Can you work these out from the model? Positions are in its coordinate system, mm. A direction names the side the tool comes from. Coordinates: 2 decimals unless noted, no trailing zeros. Order: outer loops, then holes, each group sorted by start corner. A loop starts at its lowest first (then second) coordinate and runs counter-clockwise, first axis right, second up. Notation, with made-up numbers: M -20.5,24.25 L 37.5,24.25 A28 cw 37.5,62.25 Z; hole C -13,29.25 d10. An arc over 180 degrees is marked long. Answer as CSV lines item,"result". Start each with the question number.
1. If we section it at C-C (y = -11): List the corners of the cut face in (x, z) for me, plus the area to 3 significant figures.
2. If we section it at B-B (x = 0): List the corners of the cut face in (y, z) for me.
3. If we section it at D-D (x = 18.4): List the corners of the cut face in (y, z) for me, plus the area to 3 significant figures.
4. I need wall thicknesses on line 1 along Z through (x, y) = (0, -6.15); line 2 along X through (y, z) = (-5.75, 5.25); line 3 along Y through (x, z) = (-18.5, 5). Which ranges of each line are inside material? Lowest first, please. Write a range as from..to.
5. Will these pins go through, and if not, where does the flat tip stop? pin 1 (6 mm diameter, centred on x = -18.4, z = 0, fed in from -Y); pin 2 (10.5 mm diameter, centred on x = 15, z = 4, fed in from -Y); pin 3 (4.5 mm diameter, centred on x = 18.4, z = 0, fed in from -Y); pin 4 (1 mm diameter, centred on y = -3.5, z = 1.5, fed in from -X).
6. If we section it at A-A (y = -6): List the corners of the cut face in (x, z) for me.
7. If we mould it in two halves opening along X, with no side actions, what happens to faces 3 (the face through (8.44, -8.2, -8.44)), 4 (the face through (13.4, -3.9, 0.1)), 5 (the face through (13.34, -2.071, 8.245))? For each: released by +X, released by -X, zero draft, split by the parting line, or undercut.
8. On a 3-axis mill with a long thin cutter (end or side, diameter ignored), from which of +Z, -Z, +X, -X, +Y, -Y can I reach the whole of each face in a straight line? I mean faces 1 (the face through (5.19, -5.93, -9.98)), 2 (the face through (-21, -2, 0)). Say none if no direction works.
```python
from build123d import *

# Parameters (mm, degrees)
F0_R     = 2.6
F0_R_2   = 4
F1_DEPTH = 4.2
F2_R     = 14.25
F2_R_2   = 13.25
F3_DEPTH = 0.3
F4_R     = 6.2
F4_R_2   = 4
F5_DEPTH = 7.8
F4_R_3   = 11.25
F6_DEPTH = 4
F7_SIZE  = 0.5


with BuildPart() as f1:
    # F0 (on Front) → F1 (new body)
    with BuildSketch(Plane.XZ):
        with BuildLine():
            ThreePointArc((-5.796875, -11.9146439407), (-13.25, 0), (-5.796875, 11.9146439407))
            Line((-5.796875, 11.9146439407), (-20.675, 4.6759357352))
            ThreePointArc((-20.675, 4.6759357352), (-23.6, 0), (-20.675, -4.6759357352))
            Line((-20.675, -4.6759357352), (-5.796875, -11.9146439407))
        make_face()
        with Locations((-18.4, 0)):
            Circle(F0_R, mode=Mode.SUBTRACT)
        with BuildLine():
            ThreePointArc((5.796875, -11.9146439407), (11.2332340346, -7.026873638), (13.25, 0))
            ThreePointArc((13.25, 0), (11.2332340346, 7.026873638), (5.796875, 11.9146439407))
            ThreePointArc((5.796875, 11.9146439407), (0, 13.25), (-5.796875, 11.9146439407))
            ThreePointArc((-5.796875, 11.9146439407), (-13.25, 0), (-5.796875, -11.9146439407))
            ThreePointArc((-5.796875, -11.9146439407), (0, -13.25), (5.796875, -11.9146439407))
        make_face()
        Circle(F0_R_2, mode=Mode.SUBTRACT)
        with BuildLine():
            ThreePointArc((5.796875, 11.9146439407), (11.2332340346, 7.026873638), (13.25, 0))
            ThreePointArc((13.25, 0), (11.2332340346, -7.026873638), (5.796875, -11.9146439407))
            Line((5.796875, -11.9146439407), (20.675, -4.6759357352))
            ThreePointArc((20.675, -4.6759357352), (23.6, 0), (20.675, 4.6759357352))
            Line((20.675, 4.6759357352), (5.796875, 11.9146439407))
        make_face()
        with Locations((18.4, 0)):
            Circle(F0_R, mode=Mode.SUBTRACT)
    extrude(amount=F1_DEPTH)

    # F2 (on face) → F3 (cut)
    with BuildSketch(Plane.XZ.offset(4.2)):
        Circle(F2_R)
        Circle(F2_R_2, mode=Mode.SUBTRACT)
    extrude(amount=-F3_DEPTH, mode=Mode.SUBTRACT)

    # F4 (on face) → F5 (join)
    with BuildSketch(Plane.XZ.offset(4.2)):
        Circle(F4_R)
        Circle(F4_R_2, mode=Mode.SUBTRACT)
    extrude(amount=F5_DEPTH)

    # F4 (on face) → F6 (join)
    with BuildSketch(Plane.XZ.offset(4.2)):
        with BuildLine():
            ThreePointArc((5.796875, -11.9146439407), (11.2332340346, -7.026873638), (13.25, 0))
            ThreePointArc((13.25, 0), (11.2332340346, 7.026873638), (5.796875, 11.9146439407))
            ThreePointArc((5.796875, 11.9146439407), (0, 13.25), (-5.796875, 11.9146439407))
            ThreePointArc((-5.796875, 11.9146439407), (-13.25, 0), (-5.796875, -11.9146439407))
            ThreePointArc((-5.796875, -11.9146439407), (0, -13.25), (5.796875, -11.9146439407))
        make_face()
        Circle(F4_R_3, mode=Mode.SUBTRACT)
    extrude(amount=F6_DEPTH)

    # F7
    f7_edges = [f1.edges().sort_by_distance(p)[0] for p in [
        (-4, -12, 0),
        (-6.2, -12, 0),
        (-11.25, -8.2, 0),
        (5.796875, -8.2, -11.914644),
    ]]
    chamfer(f7_edges, length=F7_SIZE)


solid = f1.part
```
Solved:
1,outline,"C 0,0 d12.4; hole C 0,0 d8"
1,area,"70.5 mm²"
2,outline,"M -12,-5.7 L -11.5,-6.2 L -4.2,-6.2 L -4.2,-11.25 L -7.7,-11.25 L -8.2,-11.75 L -8.2,-12.75 L -7.7,-13.25 L 0,-13.25 L 0,-4 L -11.5,-4 L -12,-4.5 Z; M -12,4.5 L -11.5,4 L 0,4 L 0,13.25 L -7.7,13.25 L -8.2,12.75 L -8.2,11.75 L -7.7,11.25 L -4.2,11.25 L -4.2,6.2 L -11.5,6.2 L -12,5.7 Z"
3,outline,"M -4.2,-5.78 L 0,-5.78 L 0,-2.6 L -4.2,-2.6 Z; M -4.2,2.6 L 0,2.6 L 0,5.78 L -4.2,5.78 Z"
3,area,"26.7 mm²"
4,line 1,"-13.25..-11.25, -6.2..-4, 4..6.2, 11.25..13.25"
4,line 2,"-12.17..-9.95, -3.3..3.3, 9.95..12.17"
4,line 3,"-4.2..0"
5,pin 1,"y = -4.2"
5,pin 2,"y = -8.2"
5,pin 3,"through"
5,pin 4,"x = -23.5"
6,outline,"C 0,0 d26.5; C 0,0 d12.4; hole C 0,0 d22.5; hole C 0,0 d8"
7,face 3,"zero draft"
7,face 4,"undercut"
7,face 5,"released by +X"
8,face 1,"-Y"
8,face 2,"+Y, -Y"
